For this review, take the finished solid that the model builds, in its own axes (mm). A direction names the side the tool comes from. Coordinates: 2 decimals unless noted, no trailing zeros. Loops run counter-clockwise (first coordinate to the right, second up) from the corner with the lowest first, then second, coordinate; pieces in that order, holes last.
1. Machinability: for faces 1 (the face through (38, -17, 4)), 2 (the face through (24, -8, 13)), 3 (the face through (41.93, 10.6, 4.56)), 4 (the face through (21.118, 0, 28)), 5 (the face through (14.5, -24, 13)), which of the approach directions +Z, -Z, +X, -X, +Y, -Y give a long, thin tool a straight path to every point of the face, cutting with its end or side? Answer none if there is none.
2. Clearance check with flat-ended pins moving along their axes: P1, Ø7, axis at x = 29, z = 5, coming from the -Y side; P2, Ø3, axis at x = 29.5, z = 28, coming from the +Y side; P3, Ø5, axis at x = 24, z = 21, coming from the -Y side; P4, Ø4.5, axis at x = -36, z = 6.5, coming from the -Y side. State where each tip first meets the part, or that it passes through.
3. Take a section at A-A, the plane x = -35. State the section outline as (y, z) points, then the cut area to 3 significant figures.
4. Take a section at B-B, the plane y = -4. State the section outline as (x, z) points, then the cut area to 3 significant figures.
5. Take a section at D-D, the plane x = 12.5. State the section outline as (y, z) points, then the cut area to 3 significant figures.
6. To check wall thickness, follow probe 1 along Y at (x, z) = (35, 7.7); probe 2 along Y at (x, z) = (35, 1); probe 3 along Y at (x, z) = (-35, 1.9). State the ranges of each line that lie inside material, in increasing order.
7. Take a section at C-C, the plane z = 19.5. Count the separate pieces of the cut face and the enclosed holes in it, then the cut area to 3 significant figures.
8. Mouldability with a two-part tool opening along Y and no side actions: class faces 6 (the face through (36.916, 19.257, 1.972)), 7 (the face through (-41.9, 10.57, 4.56)), 8 (the face through (-26, 18, 0)) as pulls with the +Y half, pulls with the -Y half, needs draft (parallel to the pull), parting line crosses it, or undercut.
```python
from build123d import *

# Parameters (mm, degrees)
SKETCH2_W           = 55
SKETCH2_H           = 55
BOSS_EXTRUDE1_DEPTH = 33.6
BOSS_EXTRUDE2_DEPTH = 3
SKETCH4_W           = 15
SKETCH4_H           = 15
SKETCH4_R           = 2.6
BOSS_EXTRUDE3_DEPTH = 9
CUT_EXTRUDE1_START  = -5
SKETCH6_R           = 4.4
SKETCH6_R_2         = 2.6
CUT_EXTRUDE1_DEPTH  = 5
CHAMFER1_SIZE       = 5
FILLET4_R           = 2
SKETCH7_W           = 24
SKETCH7_H           = 26.6
CUT_EXTRUDE2_DEPTH  = 67
SKETCH8_W           = 26.6
SKETCH8_H           = 16
CUT_EXTRUDE3_DEPTH  = 67


with BuildPart() as part:
    # Sketch2 → Boss-Extrude1 (new body)
    with BuildSketch(Plane.XY):
        with Locations((0, 0.476186899)):
            Rectangle(SKETCH2_W, SKETCH2_H)
        Polygon((21.118377871, -17.280631787), (21.118377871, 17.280631787), (17.280631787, 21.118377871), (-17.280631787, 21.118377871), (-21.118377871, 17.280631787), (-21.118377871, -17.280631787), (-17.280631787, -21.118377871), (17.280631787, -21.118377871), align=None, mode=Mode.SUBTRACT)
    extrude(amount=BOSS_EXTRUDE1_DEPTH)

    # Sketch3 → Boss-Extrude2 (add)
    with BuildSketch(Plane.XY.offset(33.6)):
        with BuildLine():
            Line((-7.954951288, 8.431138187), (-18.961411379, 19.437598278))
            Line((-18.961411379, 19.437598278), (-21.118377871, 17.280631787))
            Line((-21.118377871, 17.280631787), (-21.118377871, -17.280631787))
            Line((-21.118377871, -17.280631787), (-19.437598278, -18.961411379))
            Line((-19.437598278, -18.961411379), (-7.954951288, -7.478764389))
            ThreePointArc((-7.954951288, -7.478764389), (-11.25, 0.476186899), (-7.954951288, 8.431138187))
        make_face()
        with BuildLine():
            Line((-7.954951288, -7.478764389), (-19.437598278, -18.961411379))
            Line((-19.437598278, -18.961411379), (-17.280631787, -21.118377871))
            Line((-17.280631787, -21.118377871), (17.280631787, -21.118377871))
            Line((17.280631787, -21.118377871), (19.437598278, -18.961411379))
            Line((19.437598278, -18.961411379), (7.954951288, -7.478764389))
            ThreePointArc((7.954951288, -7.478764389), (0, -10.773813101), (-7.954951288, -7.478764389))
        make_face()
        with BuildLine():
            Line((21.118377871, 17.280631787), (18.961411379, 19.437598278))
            Line((18.961411379, 19.437598278), (7.954951288, 8.431138187))
            ThreePointArc((7.954951288, 8.431138187), (10.393644741, 4.781375513), (11.25, 0.476186899))
            ThreePointArc((11.25, 0.476186899), (10.393644741, -3.829001715), (7.954951288, -7.478764389))
            Line((7.954951288, -7.478764389), (19.437598278, -18.961411379))
            Line((19.437598278, -18.961411379), (21.118377871, -17.280631787))
            Line((21.118377871, -17.280631787), (21.118377871, 17.280631787))
        make_face()
        with BuildLine():
            Line((-17.280631787, 21.118377871), (-18.961411379, 19.437598278))
            Line((-18.961411379, 19.437598278), (-7.954951288, 8.431138187))
            ThreePointArc((-7.954951288, 8.431138187), (0, 11.726186899), (7.954951288, 8.431138187))
            Line((7.954951288, 8.431138187), (18.961411379, 19.437598278))
            Line((18.961411379, 19.437598278), (17.280631787, 21.118377871))
            Line((17.280631787, 21.118377871), (-17.280631787, 21.118377871))
        make_face()
        Polygon((-18.961411379, 19.437598278), (-27.5, 27.976186899), (-27.5, -27.023813101), (-19.437598278, -18.961411379), (-21.118377871, -17.280631787), (-21.118377871, 17.280631787), align=None)
        Polygon((-19.437598278, -18.961411379), (-27.5, -27.023813101), (27.5, -27.023813101), (19.437598278, -18.961411379), (17.280631787, -21.118377871), (-17.280631787, -21.118377871), align=None)
        Polygon((27.5, -27.023813101), (27.5, 27.976186899), (18.961411379, 19.437598278), (21.118377871, 17.280631787), (21.118377871, -17.280631787), (19.437598278, -18.961411379), align=None)
        Polygon((27.5, 27.976186899), (-27.5, 27.976186899), (-18.961411379, 19.437598278), (-17.280631787, 21.118377871), (17.280631787, 21.118377871), (18.961411379, 19.437598278), align=None)
    extrude(amount=BOSS_EXTRUDE2_DEPTH)

    # Sketch4 → Boss-Extrude3 (add)
    # profile 1 of 4: a face of its own
    with BuildSketch(Plane(origin=(0, 0, 0), x_dir=(-1, 0, 0), z_dir=(0, 0, -1))):
        with Locations((-35, 17.5)):
            Rectangle(SKETCH4_W, SKETCH4_H)
        with Locations((-35, 17.5)):
            Circle(SKETCH4_R, mode=Mode.SUBTRACT)
    # profile 2 of 4: a face of its own
    with BuildSketch(Plane(origin=(0, 0, 0), x_dir=(-1, 0, 0), z_dir=(0, 0, -1))):
        with Locations((35, 17.5)):
            Rectangle(SKETCH4_W, SKETCH4_H)
        with Locations((35, 17.5)):
            Circle(SKETCH4_R, mode=Mode.SUBTRACT)
    # profile 3 of 4: a face of its own
    with BuildSketch(Plane(origin=(0, 0, 0), x_dir=(-1, 0, 0), z_dir=(0, 0, -1))):
        with Locations((-35, -17.5)):
            Rectangle(SKETCH4_W, SKETCH4_H)
        with Locations((-35, -17.5)):
            Circle(SKETCH4_R, mode=Mode.SUBTRACT)
    # profile 4 of 4: a face of its own
    with BuildSketch(Plane(origin=(0, 0, 0), x_dir=(-1, 0, 0), z_dir=(0, 0, -1))):
        with Locations((17.5, -34.523813101)):
            Rectangle(SKETCH4_W, SKETCH4_H)
        with Locations((17.5, -34.523813101)):
            Circle(SKETCH4_R, mode=Mode.SUBTRACT)
    extrude(amount=-BOSS_EXTRUDE3_DEPTH)

    # Sketch6 → Cut-Extrude1 (cut)
    # profile 1 of 4: a face of its own
    with BuildSketch(Plane.XY.offset(9).offset(CUT_EXTRUDE1_START)):
        with Locations((-17.5, -34.523813101)):
            Circle(SKETCH6_R)
    # profile 2 of 4: a face of its own
    with BuildSketch(Plane.XY.offset(9).offset(CUT_EXTRUDE1_START)):
        with Locations((-35, 17.5)):
            Circle(SKETCH6_R)
    # profile 3 of 4: a face of its own
    with BuildSketch(Plane.XY.offset(9).offset(CUT_EXTRUDE1_START)):
        with Locations((35, -17.5)):
            Circle(SKETCH6_R)
        with Locations(Location((35, -17.5, 0), (0, 0, 180))):
            Circle(SKETCH6_R_2, mode=Mode.SUBTRACT)
    # profile 4 of 4: a face of its own
    with BuildSketch(Plane.XY.offset(9).offset(CUT_EXTRUDE1_START)):
        with Locations((35, 17.5)):
            Circle(SKETCH6_R)
    extrude(amount=CUT_EXTRUDE1_DEPTH, mode=Mode.SUBTRACT)

    # Chamfer1
    chamfer1_edges = [part.edges().sort_by_distance(p)[0] for p in [
        (27.5, -27.023813101, 18.3),
        (-27.5, -27.023813101, 18.3),
        (27.5, 27.976186899, 18.3),
        (-27.5, 27.976186899, 18.3),
    ]]
    chamfer(chamfer1_edges, length=CHAMFER1_SIZE)

    # Fillet4
    fillet4_edges = [part.edges().sort_by_distance(p)[0] for p in [
        (0, 27.976186899, 36.6),
        (27.5, 0.476186899, 36.6),
        (0, -27.023813101, 36.6),
        (-27.5, 0.476186899, 36.6),
        (-25, -42.023813101, 4.5),
        (-10, -42.023813101, 4.5),
        (-42.5, 10, 4.5),
        (-42.5, 25, 4.5),
        (42.5, -25, 4.5),
        (42.5, -10, 4.5),
        (42.5, 10, 4.5),
        (42.5, 25, 4.5),
    ]]
    fillet(fillet4_edges, radius=FILLET4_R)

    # Sketch7 → Cut-Extrude2 (cut)
    with BuildSketch(Plane.XZ.offset(27.023813101)):
        with Locations((2.5, 13.3)):
            Rectangle(SKETCH7_W, SKETCH7_H)
    extrude(amount=-CUT_EXTRUDE2_DEPTH, mode=Mode.SUBTRACT)

    # Sketch8 → Cut-Extrude3 (cut)
    with BuildSketch(Plane.ZY.offset(27.5)):
        with Locations((13.3, 0)):
            Rectangle(SKETCH8_W, SKETCH8_H)
    extrude(amount=-CUT_EXTRUDE3_DEPTH, mode=Mode.SUBTRACT)


solid = part.part
```
Results list:
1. face 1: +Z
1. face 2: -Z, +X, -X
1. face 3: +Z, -Z, +X
1. face 4: -Z
1. face 5: -Z, +Y, -Y
2. P1: stops at y = -25
2. P2: passes through
2. P3: stops at y = -27.02
2. P4: stops at y = 10
3. outline: (10, 0) - (14.9, 0) - (14.9, 4) - (13.1, 4) - (13.1, 9) - (10, 9) - close; (20.1, 0) - (25, 0) - (25, 9) - (21.9, 9) - (21.9, 4) - (20.1, 4) - close
3. area: 70.2 mm2
4. outline: (-27.5, 26.6) - (-21.12, 26.6) - (-21.12, 33.6) - (-10.32, 33.6) - (-10.32, 36.6) - (-25.5, 36.6) arc R2 ccw to (-27.5, 34.6) - close; (10.32, 33.6) - (21.12, 33.6) - (21.12, 26.6) - (27.5, 26.6) - (27.5, 34.6) arc R2 ccw to (25.5, 36.6) - (10.32, 36.6) - close
4. area: 191 mm2
5. outline: (-27.02, 26.6) - (-21.12, 26.6) - (-21.12, 33.6) - (21.12, 33.6) - (21.12, 26.6) - (27.98, 26.6) - (27.98, 34.6) arc R2 ccw to (25.98, 36.6) - (-25.02, 36.6) arc R2 ccw to (-27.02, 34.6) - close
5. area: 253 mm2
6. probe 1: y = -25 to -21.9, -13.1 to -10, 10 to 13.1, 21.9 to 25
6. probe 2: y = -25 to -20.1, -14.9 to -10, 10 to 14.9, 20.1 to 25
6. probe 3: y = 10 to 14.9, 20.1 to 25
7. separate pieces: 4
7. enclosed holes: 0
7. area: 710 mm2
8. face 6: undercut
8. face 7: pulls with the -Y half
8. face 8: needs draft
